Source: CAD feature listing. Evaluate the final solid. Frame: model axes, mm. Face numbers are marked on the shaded views. A direction names the side the tool comes from. Give positions to 0.01 mm unless a question says otherwise; leave off trailing zeros. Loops run counter-clockwise (first coordinate to the right, second up) from the corner with the lowest first, then second, coordinate; pieces in that order, holes last.
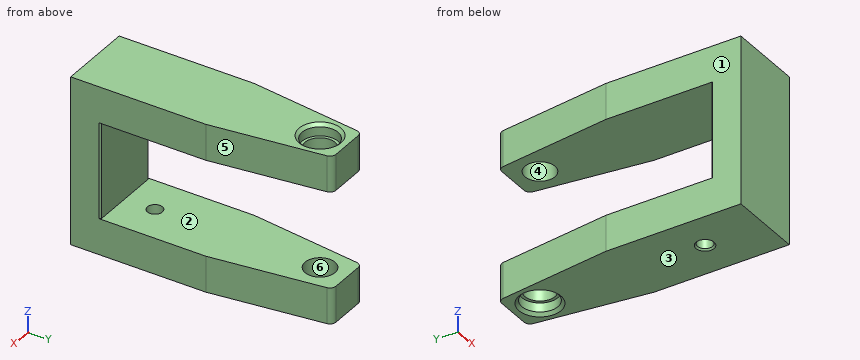
from build123d import *

# Parameters (mm, degrees)
BOSS_EXTRUDE1_DEPTH         = 28
SKETCH2_W                   = 32
SKETCH2_H                   = 74
CUT_EXTRUDE1_DEPTH          = 56
FILLET1_R                   = 2
CHAMFER1_SIZE               = 0.5
M6_TAPPED_HOLE2_D           = 5
M6_TAPPED_HOLE2_DEPTH       = 27
M6_TAPPED_HOLE2_CSINK_D     = 6.05
M6_TAPPED_HOLE2_CSINK_ANGLE = 90
M6_TAPPED_HOLE2_TIP         = 1.502151548


with BuildPart() as part:
    # Sketch1 → Boss-Extrude1 (new, symmetric)
    with BuildSketch(Plane.XY):
        Polygon((12.5, 0), (-12.5, 0), (-12.5, 45), (-7.5, 84), (7.5, 84), (12.5, 45), align=None)
    extrude(amount=BOSS_EXTRUDE1_DEPTH, both=True)

    # Sketch2 → Cut-Extrude1 (cut)
    with BuildSketch(Plane(origin=(12.5, 0, 0), x_dir=(0, 0, -1), z_dir=(1, 0, 0))):
        with Locations((0, 47)):
            Rectangle(SKETCH2_W, SKETCH2_H)
    extrude(amount=-CUT_EXTRUDE1_DEPTH, mode=Mode.SUBTRACT)

    # Sketch4 → CBORE for M4 Hex Socket Head Cap Screw1 (revolve, cut)
    with BuildSketch(Plane(origin=(0, 75, -28), x_dir=(0, 1, 0), z_dir=(1, 0, 0))):
        Polygon((0, 0), (0, 23.004303095), (5, 20), (5, 4), (6, 4), (6, 1), (7, 0), align=None)
    cbore_for_m4_hex_socket_head_cap_screw1 = revolve(axis=Axis((0, 75, -34.35), (0, 0, 1)), mode=Mode.SUBTRACT)

    # Mirror1: CBORE for M4 Hex Socket Head Cap Screw1 across plane
    add(cbore_for_m4_hex_socket_head_cap_screw1.mirror(Plane.XY), mode=Mode.SUBTRACT)

    # Fillet1
    fillet1_edges = [part.edges().sort_by_distance(p)[0] for p in [
        (-7.5, 84, 22),
        (7.5, 84, 22),
        (-7.5, 84, -22),
        (7.5, 84, -22),
    ]]
    fillet(fillet1_edges, radius=FILLET1_R)

    # Chamfer1
    chamfer1_edges = [part.edges().sort_by_distance(p)[0] for p in [
        (-12.5, 10, 0),
        (12.5, 10, 0),
    ]]
    chamfer(chamfer1_edges, length=CHAMFER1_SIZE)

    # M6 Tapped Hole2
    with Locations(Plane(origin=(0, 0, -28), x_dir=(-1, 0, 0), z_dir=(0, 0, -1))):
        with Locations((0, 20)):
            CounterSinkHole(M6_TAPPED_HOLE2_D / 2, M6_TAPPED_HOLE2_CSINK_D / 2, depth=M6_TAPPED_HOLE2_DEPTH, counter_sink_angle=M6_TAPPED_HOLE2_CSINK_ANGLE)
            with Locations((0, 0, -(M6_TAPPED_HOLE2_DEPTH + M6_TAPPED_HOLE2_TIP / 2))):  # 118° drill point
                Cone(0, M6_TAPPED_HOLE2_D / 2, M6_TAPPED_HOLE2_TIP, mode=Mode.SUBTRACT)


solid = part.part
1) Ray query, probe 1 along Z at (x, y) = (5, 36); probe 2 along Y at (x, z) = (0, 24.9); probe 3 along Y at (x, z) = (-4, -25). Return the intervals inside material, ascending.
Checks:
probe 1: z = -28 to -16, 16 to 28
probe 2: y = 0 to 69, 81 to 84
probe 3: y = 0 to 70.53, 79.47 to 84
2) Cut plane A-A (y = 44). Return loops of the section in (x, z).
Checks:
outline: (-12.5, -28) - (12.5, -28) - (12.5, -16) - (-12.5, -16) - close; (-12.5, 16) - (12.5, 16) - (12.5, 28) - (-12.5, 28) - close
3) Contact query for flat-ended pins moving along their axis: P1, Ø7, axis at x = 0, y = 75, coming from the -Z side; P2, Ø1.5, axis at x = 1.5, z = -11.5, coming from the +Y side; P3, Ø10, axis at x = -2.5, z = 2, coming from the -Y side; P4, Ø4, axis at x = 0, y = 20, coming from the -Z side. Output: stop coordinate, or through.
Checks:
P1: passes through
P2: stops at y = 10
P3: stops at y = 0
P4: stops at z = 16
4) Reachability of the marked faces 1 and 2 from +Z, -Z, +X, -X, +Y, -Y: full face, straight path, thin tool, end or side. Return the list, or none.
Checks:
face 1: +Z, -Z, -X, +Y, -Y
face 2: +X, -X, +Y
5) Cut plane D-D (z = -19.5). Return loops of the section in (x, y).
Checks:
outline: (-12.5, 0) - (12.5, 0) - (12.5, 45) - (7.72, 82.25) arc R2 ccw to (5.74, 84) - (-5.74, 84) arc R2 ccw to (-7.72, 82.25) - (-12.5, 45) - close; hole circle Ø10 at (0, 75); hole circle Ø5 at (0, 20)
6) Cut plane B-B (x = 0). State how many separate pieces and enclosed holes the cut face has, and give its area (3 significant figures).
Checks:
separate pieces: 4
enclosed holes: 0
area: 2,020 mm2
7) Cut plane C-C (z = 22.5). Return loops of the section in (x, y), and give its area (3 significant figures).
Checks:
outline: (-12.5, 0) - (12.5, 0) - (12.5, 45) - (7.72, 82.25) arc R2 ccw to (5.74, 84) - (-5.74, 84) arc R2 ccw to (-7.72, 82.25) - (-12.5, 45) - close; hole circle Ø10 at (0, 75)
area: 1,830 mm2
8) Pull-direction query (Y, two-part tool) for the marked faces 3, 4, 5 and 6; classes: released by +Y, released by -Y, zero draft, split by the parting line, or undercut.
Checks:
face 3: zero draft
face 4: undercut
face 5: released by +Y
face 6: undercut
